Verification items for the finished model (mm, model axes). Face numbers are marked on the shaded views. A direction names the side the tool comes from. Coordinates: 2 decimals unless noted, no trailing zeros. Write each loop counter-clockwise with the first axis right and the second up, starting at its lowest first coordinate (ties: lowest second). Pieces come first, ordered by that corner, then holes.
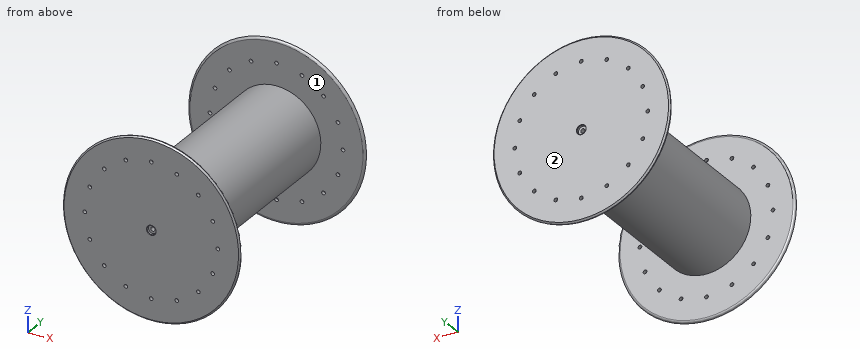
```python
from build123d import *

# Parameters (mm, degrees)
SKETCH1_R                = 60
BOSS_EXTRUDE1_DEPTH      = 140
SKETCH3_R                = 120
BOSS_EXTRUDE2_DEPTH      = 5
CHAMFER1_SIZE            = 2
FILLET1_R                = 3
CHAMFER1_OF_MIRROR8_SIZE = 2
FILLET1_OF_MIRROR8_R     = 3
SKETCH4_R                = 2.5
CUT_EXTRUDE1_DEPTH       = 337.005952328
CIRPATTERN1_COUNT        = 16


with BuildPart() as part:
    # Sketch1 → Boss-Extrude1 (new, symmetric)
    with BuildSketch(Plane(origin=(0, 0, 0), x_dir=(1, 0, 0), z_dir=(0, 1, 0))):
        with Locations(Location((0, 0, 0), (0, 0, 270))):
            Circle(SKETCH1_R)
    extrude(amount=BOSS_EXTRUDE1_DEPTH, both=True)

    # Sketch3 → Boss-Extrude2 (add)
    with BuildSketch(Plane(origin=(0, 140, 0), x_dir=(1, 0, 0), z_dir=(0, 1, 0))):
        with Locations(Location((0, 0, 0), (0, 0, 270))):
            Circle(SKETCH3_R)
    boss_extrude2 = extrude(amount=BOSS_EXTRUDE2_DEPTH)

    # Chamfer1
    chamfer1_edges = [part.edges().sort_by_distance(p)[0] for p in [
        (0, 145, -120),
    ]]
    chamfer(chamfer1_edges, length=CHAMFER1_SIZE)

    # Fillet1
    fillet1_edges = [part.edges().sort_by_distance(p)[0] for p in [
        (0, 140, -120),
    ]]
    fillet(fillet1_edges, radius=FILLET1_R - 0.0001)  # a hair under: the kernel refuses the full size

    # Sketch8 → CBORE for #12 Binding Head Machine Screw2 (revolve, cut)
    with BuildSketch(Plane(origin=(0, 145, 0), x_dir=(0, 0, 1), z_dir=(1, 0, 0))):
        Polygon((0, 0), (0, 290), (2.8956, 290), (2.8956, 3.5814), (5.95376, 3.5814), (5.95376, 0.635), (6.58876, 0), align=None)
    cbore_for_12_binding_head_machine_screw = revolve(axis=Axis((0, 151.35, 0), (0, -1, 0)), mode=Mode.SUBTRACT)

    # Mirror8: Boss-Extrude2, CBORE for #12 Binding Head Machine Screw2 across plane
    add(boss_extrude2.mirror(Plane.ZX))
    add(cbore_for_12_binding_head_machine_screw.mirror(Plane.ZX), mode=Mode.SUBTRACT)

    # Chamfer1 of Mirror8
    chamfer1_of_mirror8_edges = [part.edges().sort_by_distance(p)[0] for p in [
        (0, -145, -120),
    ]]
    chamfer(chamfer1_of_mirror8_edges, length=CHAMFER1_OF_MIRROR8_SIZE)

    # Fillet1 of Mirror8
    fillet1_of_mirror8_edges = [part.edges().sort_by_distance(p)[0] for p in [
        (0, -140, -120),
    ]]
    fillet(fillet1_of_mirror8_edges, radius=FILLET1_OF_MIRROR8_R - 0.0001)  # a hair under: the kernel refuses the full size

    # Sketch4 → Cut-Extrude1 (cut, symmetric)
    with BuildSketch(Plane(origin=(0, 145, 0), x_dir=(1, 0, 0), z_dir=(0, 1, 0))):
        with Locations(Location((0, 90, 0), (0, 0, 270))):
            Circle(SKETCH4_R)
    cut_extrude1 = extrude(amount=CUT_EXTRUDE1_DEPTH, both=True, mode=Mode.SUBTRACT)

    # CirPattern1: Cut-Extrude1 ×16 about axis
    cirpattern1_axis = Axis((0, 0, 0), (0, 1, 0))
    for i in range(1, CIRPATTERN1_COUNT):
        add(cut_extrude1.rotate(cirpattern1_axis, i * 360 / CIRPATTERN1_COUNT), mode=Mode.SUBTRACT)


solid = part.part
```
1. Tool access check on the marked faces 1 and 2. Record the directions out of +Z, -Z, +X, -X, +Y, -Y that give a thin tool (end or side, any length) a straight path to the whole face; none if there is none.
2. Material ranges on L1, parallel to Y at x = -44, z = 69.5; L2, parallel to Z at x = -90, y = 143; L3, parallel to X at y = 141, z = -90, recorded low to high.
3. Sectioned sample at A-A, the plane y = -111. Record the boundary of the cut face in (x, z).
4. Gauge pin test, flat ends, axial feed: P1, Ø4, axis at x = 34.44, z = 83.15, coming from the +Y side; P2, Ø3, axis at x = -41.5, y = -36.5, coming from the -Z side; P3, Ø1.5, axis at x = 53, y = 44.5, coming from the +Z side; P4, Ø3, axis at y = 50, z = 6.5, coming from the -X side. Record the tip position at first contact, or that the pin passes through.
Outcome:
1. face 1: none
1. face 2: +Z, -Z, +X, -X, +Y
2. L1: y = -145 to -140, 140 to 145
2. L2: z = -79.37 to -2.5, 2.5 to 79.37
2. L3: x = -78.21 to -2.5, 2.5 to 78.21
3. outline: circle Ø120 at (0, 0); hole circle Ø5.79 at (0, 0)
4. P1: passes through
4. P2: stops at z = -44.72
4. P3: stops at z = 29.49
4. P4: stops at x = -59.79
